Can you work these out from the drawing? Everything is in mm from the part's minimum corner. Coordinates: 2 decimals unless noted, no trailing zeros. Order: outer loops, then holes, each group sorted by start corner. A loop starts at its lowest first (then second) coordinate and runs counter-clockwise, first axis right, second up. Notation, with made-up numbers: (62, 83.5) -> (85, 83.5) arc R34 ccw to (85, 114.5) -> close; hole circle Ø11 at (-39.75, -36). An arc over 180 degrees is marked (long way). Put each result on its own line as item: value. Start each with the question number.
Q1. Please list where these lines run through material, in increasing order: line 1 along X through (y, z) = (1.45, 5) (3 decimals); line 2 along X through (y, z) = (2.3, 6); line 3 along X through (y, z) = (1.7, 17.9) (3 decimals).
Q2. If we section it at A-A (z = 35.9): Please give me the cut outline in (x, y) (3 decimals), and give its area (4 significant figures).
Q3. Will these pins go through, and if not, where does the flat tip stop? pin 1 (1.5 mm diameter, centred on x = 13.5, y = 1, fed in from +Z); pin 2 (1.5 mm diameter, centred on y = 1.5, z = 26, fed in from +X).
Q4. If we section it at B-B (y = 2): Please give me the cut outline in (x, z) (3 decimals).
Q5. If we section it at D-D (z = 5): Please give me the cut outline in (x, y) (3 decimals), and give its area (3 significant figures).
Q6. If we section it at C-C (x = 15): Please give me the cut outline in (y, z) (3 decimals).
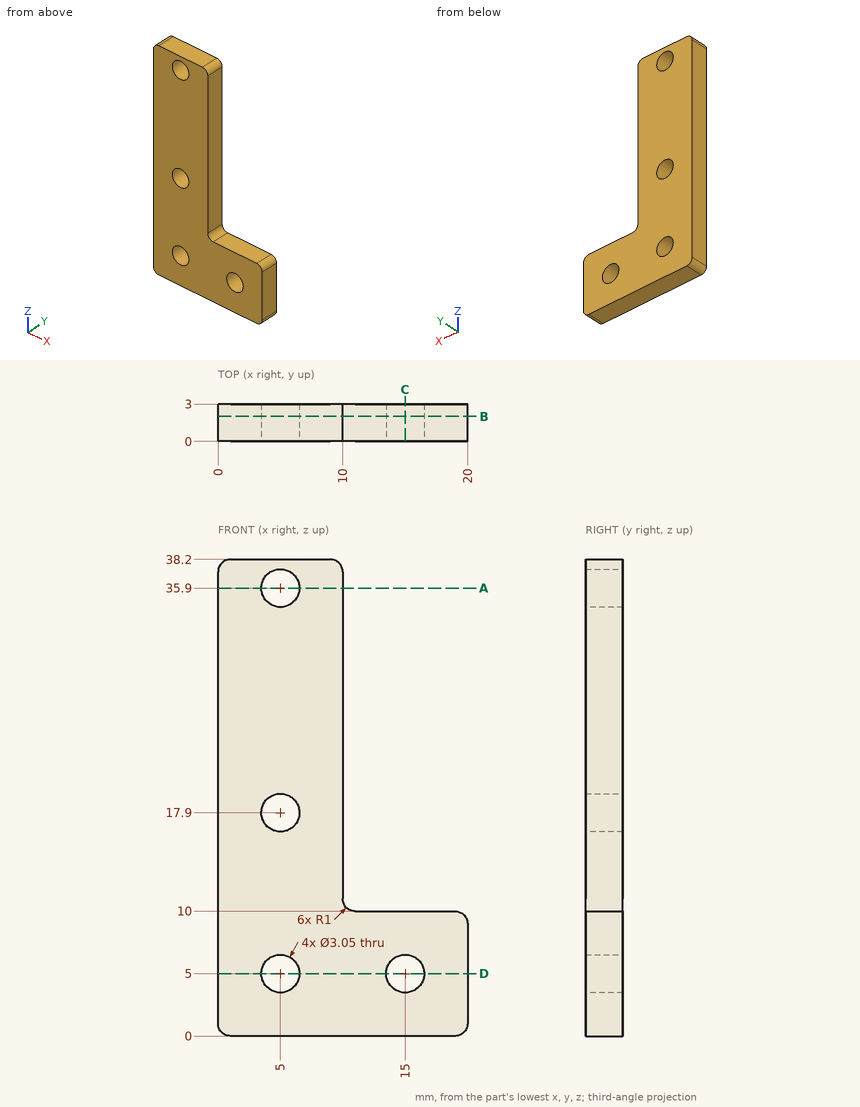
The answers:
1. line 1: 0 to 3.475, 6.525 to 13.475, 16.525 to 20
1. line 2: 0 to 3.85, 6.15 to 13.85, 16.15 to 20
1. line 3: 0 to 3.475, 6.525 to 10
2. outline: (0, 0) -> (3.475, 0) -> (3.475, 3) -> (0, 3) -> close; (6.525, 0) -> (10, 0) -> (10, 3) -> (6.525, 3) -> close
2. area: 20.85 mm^2
3. pin 1: z = 10
3. pin 2: x = 10
4. outline: (0, 1) arc R1 ccw to (1, 0) -> (19, 0) arc R1 ccw to (20, 1) -> (20, 9) arc R1 ccw to (19, 10) -> (11, 10) arc R1 cw to (10, 11) -> (10, 37.2) arc R1 ccw to (9, 38.2) -> (1, 38.2) arc R1 ccw to (0, 37.2) -> close; hole circle Ø3.05 at (5, 5); hole circle Ø3.05 at (5, 17.9); hole circle Ø3.05 at (5, 35.9); hole circle Ø3.05 at (15, 5)
5. outline: (0, 0) -> (3.475, 0) -> (3.475, 3) -> (0, 3) -> close; (6.525, 0) -> (13.475, 0) -> (13.475, 3) -> (6.525, 3) -> close; (16.525, 0) -> (20, 0) -> (20, 3) -> (16.525, 3) -> close
5. area: 41.7 mm^2
6. outline: (0, 0) -> (3, 0) -> (3, 3.475) -> (0, 3.475) -> close; (0, 6.525) -> (3, 6.525) -> (3, 10) -> (0, 10) -> close
